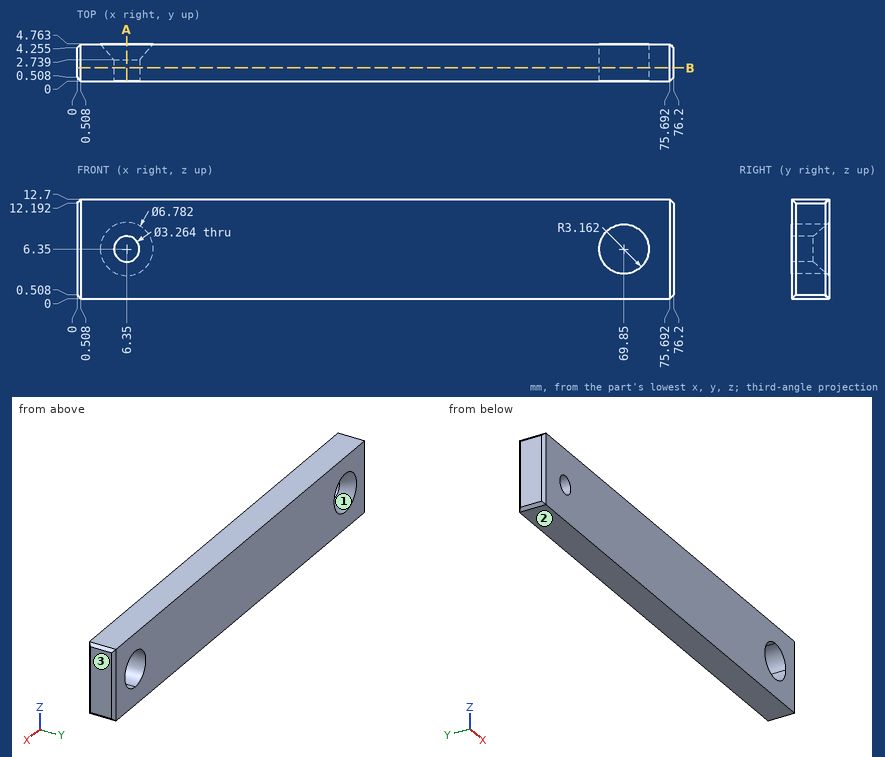
Verification items for this drawing (mm, ordinates from the low corner). Coordinates: 2 decimals unless noted, no trailing zeros. Order: outer loops, then holes, each group sorted by start corner. A loop starts at its lowest first (then second) coordinate and runs counter-clockwise, first axis right, second up. Notation, with made-up numbers: M 72,81 L 93,81 A29 ccw 93,116 Z; hole C 46,34.25 d7. An arc over 180 degrees is marked long. One line per item, written item: value. Start each with the question number.
Item 1: Sectioned sample at B-B on y = 1.7. Give the number of separate pieces and of enclosed holes in the cut face.
Item 2: Mould release check, pull along Z, two halves, no side actions. Record for the marked faces 1, 2 and 3: pulls with the +Z half, pulls with the -Z half, needs draft (parallel to the pull), parting line crosses it, or undercut.
Item 3: Thickness scan on probe 1 along X at (y, z) = (4.15, 7.75) (1 decimal); probe 2 along Z at (x, y) = (6.35, 1.9); probe 3 along X at (y, z) = (3.5, 8.25) (1 decimal). Record the ranges inside material, lowest first.
Item 4: Sectioned sample at A-A on x = 6.35. Record the cut outline in (y, z).
Item 5: Depth check by flat-ended pin: P1, Ø4, axis at x = 6.35, z = 6.35, coming from the +Y side; P2, Ø5, axis at x = 7.5, z = 5.5, coming from the +Y side. Enter the tip coordinate at first touch or a pass-through.
Calculated:
1. separate pieces: 1
1. enclosed holes: 2
2. face 1: undercut
2. face 2: pulls with the -Z half
2. face 3: needs draft
3. probe 1: 0 to 3.9, 8.8 to 67, 72.7 to 76.2
3. probe 2: 0 to 4.72, 7.98 to 12.7
3. probe 3: 0 to 5.1, 7.6 to 67.3, 72.4 to 76.2
4. outline: M 0,0 L 4.76,0 L 4.76,2.96 L 2.74,4.72 L 0,4.72 Z; M 0,7.98 L 2.74,7.98 L 4.76,9.74 L 4.76,12.7 L 0,12.7 Z
5. P1: y = 3.16
5. P2: y = 4.76
